```python
from build123d import *

# Parameters (mm, degrees)
SKETCH2_W                = 6
SKETCH2_H                = 14.5
BOSS_EXTRUDE1_DEPTH      = 5
SKETCH3_R                = 2.5
SKETCH3_R_2              = 1.8
BOSS_EXTRUDE2_DEPTH      = 2.5
CHAMFER2_SIZE            = 0.2
CHAMFER3_SIZE            = 0.2
SKETCH4_R                = 1.8
CUT_EXTRUDE1_DEPTH       = 14.02
SKETCH5_R                = 0.75
BOSS_EXTRUDE3_DEPTH      = 0.75
FILLET1_R                = 0.2
SKETCH7_W                = 0.344908333
SKETCH7_H                = 1.981698852
CUT_EXTRUDE2_DEPTH       = 12.710038429
SURFACE_EXTRUDE1_1_BACK  = 0.5
SURFACE_EXTRUDE1_1_DEPTH = 1
THICKEN1_T1              = 0.1
SKETCH9_W                = 1
SKETCH9_H                = 0.1
BOSS_EXTRUDE4_DEPTH      = 0.961518788
SURFACE_EXTRUDE2_2_BACK  = 0.5
SURFACE_EXTRUDE2_2_DEPTH = 1
THICKEN2_T2              = 0.1
SKETCH11_W               = 1.821073917
SKETCH11_H               = 5.660094607
CUT_EXTRUDE3_DEPTH       = 2


with BuildPart() as part:
    # Sketch2 → Boss-Extrude1 (new body)
    with BuildSketch(Plane(origin=(0, 0, 0), x_dir=(1, 0, 0), z_dir=(0, 1, 0))):
        Rectangle(SKETCH2_W, SKETCH2_H)
    extrude(amount=BOSS_EXTRUDE1_DEPTH)

    # Sketch3 → Boss-Extrude2 (add)
    with BuildSketch(Plane.XY.offset(7.25)):
        with Locations(Location((0, 2.5, 0), (0, 0, 270))):
            Circle(SKETCH3_R)
        with Locations((0, 2.5)):
            Circle(SKETCH3_R_2, mode=Mode.SUBTRACT)
    extrude(amount=BOSS_EXTRUDE2_DEPTH)

    # Chamfer2
    chamfer2_edges = [part.edges().sort_by_distance(p)[0] for p in [
        (0, 5, 9.75),
    ]]
    chamfer(chamfer2_edges, length=CHAMFER2_SIZE)

    # Chamfer3
    chamfer3_edges = [part.edges().sort_by_distance(p)[0] for p in [
        (-1.8, 2.5, 9.75),
    ]]
    chamfer(chamfer3_edges, length=CHAMFER3_SIZE)

    # Sketch4 → Cut-Extrude1 (cut)
    with BuildSketch(Plane.XY.offset(7.25)):
        with Locations((0, 2.5)):
            Circle(SKETCH4_R)
    extrude(amount=-CUT_EXTRUDE1_DEPTH, mode=Mode.SUBTRACT)

    # Sketch5 → Boss-Extrude3 (add)
    with BuildSketch(Plane.XZ):
        with Locations(Location((0, 4.191398765, 0), (0, 0, 90))):
            Circle(SKETCH5_R)
        with Locations(Location((0, -3.600413433, 0), (0, 0, 90))):
            Circle(SKETCH5_R)
    extrude(amount=BOSS_EXTRUDE3_DEPTH)

    # Fillet1
    fillet1_edges = [part.edges().sort_by_distance(p)[0] for p in [
        (0, -0.75, 3.441398765),
        (0, -0.75, -4.350413433),
    ]]
    fillet(fillet1_edges, radius=FILLET1_R)

    # Sketch7 → Cut-Extrude2 (cut, through all)
    with BuildSketch(Plane(origin=(0, 5, 0), x_dir=(1, 0, 0), z_dir=(0, 1, 0))):
        with Locations((2.827545834, -5.146058424)):
            Rectangle(SKETCH7_W, SKETCH7_H)
    extrude(amount=-CUT_EXTRUDE2_DEPTH, mode=Mode.SUBTRACT)

    # Surface-Extrude1: a surface, the sketch's curves swept straight by 1 mm
    with BuildLine(Plane.XY.offset(5.1).offset(-SURFACE_EXTRUDE1_1_BACK), mode=Mode.PRIVATE) as surface_extrude1_1_path:
        Line((2.555091667, 0.638024488), (2.555091667, 0.294273869))
        ThreePointArc((2.555091667, 0.294273869), (2.641282487, 0.086190821), (2.849365536, 0))
        Line((2.849365536, 0), (3.961518788, 0))
    surface_extrude1_1 = Shell.extrude(surface_extrude1_1_path.wire(), (0 * SURFACE_EXTRUDE1_1_DEPTH, 0 * SURFACE_EXTRUDE1_1_DEPTH, 1 * SURFACE_EXTRUDE1_1_DEPTH))
    add(Solid.thicken(surface_extrude1_1, THICKEN1_T1))

    # Sketch9 → Boss-Extrude4 (add)
    with BuildSketch(Plane(origin=(3, 0, 0), x_dir=(0, 0, -1), z_dir=(1, 0, 0))):
        with Locations((4.604659924, 0.05)):
            Rectangle(SKETCH9_W, SKETCH9_H)
    extrude(amount=BOSS_EXTRUDE4_DEPTH)

    # Surface-Extrude2: a surface, the sketch's curves swept straight by 1 mm
    with BuildLine(Plane.ZY.offset(-SURFACE_EXTRUDE2_2_BACK), mode=Mode.PRIVATE) as surface_extrude2_2_path:
        Line((-7.25, 2.862656565), (-7.25, 0.652010512))
        ThreePointArc((-7.25, 0.652010512), (-7.440969458, 0.190969458), (-7.902010512, 0))
        Line((-7.902010512, 0), (-9.009741204, 0))
    surface_extrude2_2 = Shell.extrude(surface_extrude2_2_path.wire(), (-1 * SURFACE_EXTRUDE2_2_DEPTH, 0 * SURFACE_EXTRUDE2_2_DEPTH, 0 * SURFACE_EXTRUDE2_2_DEPTH))
    add(Solid.thicken(surface_extrude2_2, -THICKEN2_T2))

    # Sketch11 → Cut-Extrude3 (cut)
    with BuildSketch(Plane.ZY.offset(3)):
        with Locations((3.036115989, 3.2980341)):
            Rectangle(SKETCH11_W, SKETCH11_H)
    extrude(amount=-CUT_EXTRUDE3_DEPTH, mode=Mode.SUBTRACT)


solid = part.part
```
Geometry check sheet. Reference: the model listing, model coordinates, mm. A direction names the side the tool comes from. Give positions to 0.01 mm unless a question says otherwise; leave off trailing zeros. Write each loop counter-clockwise with the first axis right and the second up, starting at its lowest first coordinate (ties: lowest second). Pieces come first, ordered by that corner, then holes.
1) Gauge pin test, flat ends, axial feed: pin 1 (1.5 mm diameter, centred on y = 1.5, z = -2, fed in from +X); pin 2 (0.5 mm diameter, centred on x = 3.5, z = 5, fed in from -Y); pin 3 (0.9 mm diameter, centred on y = 1, z = -8, fed in from -X); pin 4 (1.8 mm diameter, centred on x = 0, y = 2, fed in from +Z). Record the tip position at first contact, or that the pin passes through.
2) Section check B-B, the plane x = 3.25. Record the boundary of the cut face in (y, z).
3) Release check for a two-part mould opening along Y. For faces 1 (the flat face through (0, 5, 0)), 2 (the flat face through (0, 3, -6.77)), 3 (the flat face through (0, 2, -7.35)) record: pulls with the +Y half, pulls with the -Y half, needs draft (parallel to the pull), parting line crosses it, or undercut.
4) Access from +Z, -Z, +X, -X, +Y, -Y to the whole of each face (thin tool, end or side, straight path). Record for faces 4 (the flat face through (-2, 3, 2.126)), 5 (the cylindrical face through (0.751, 0.115, 8.384)), 6 (the flat face through (-3, 2, 0)).
5) Section check C-C, the plane y = 2.5. Record the boundary of the cut face in (x, z).
6) Section check A-A, the plane z = 2.5. Record the boundary of the cut face in (x, y).
7) Material ranges on L1, parallel to Y at x = 0, z = 3; L2, parallel to Z at x = 0, y = 2; L3, parallel to Z at x = 2.75, y = 2.9, recorded low to high.
Computed:
1. pin 1: stops at x = 3
1. pin 2: stops at y = 0
1. pin 3: passes through
1. pin 4: stops at z = -6.77
2. outline: (0, -5.1) - (0.1, -5.1) - (0.1, -4.1) - (0, -4.1) - close; (0, 4.6) - (0.1, 4.6) - (0.1, 5.6) - (0, 5.6) - close
3. face 1: pulls with the +Y half
3. face 2: undercut
3. face 3: needs draft
4. face 4: -X, +Y
4. face 5: +Z
4. face 6: +Z, -Z, -X, +Y, -Y
5. outline: (-3, -7.25) - (-0.5, -7.25) - (-0.5, -7.35) - (0.5, -7.35) - (0.5, -7.25) - (3, -7.25) - (3, 4.16) - (2.66, 4.16) - (2.66, 6.14) - (3, 6.14) - (3, 7.25) - (2.5, 7.25) - (2.5, 9.55) - (2.3, 9.75) - (2, 9.75) - (1.8, 9.55) - (1.8, -6.77) - (-1.8, -6.77) - (-1.8, 2.13) - (-3, 2.13) - close; (-3, 3.95) - (-1.8, 3.95) - (-1.8, 9.55) - (-2, 9.75) - (-2.3, 9.75) - (-2.5, 9.55) - (-2.5, 7.25) - (-3, 7.25) - close
6. outline: (-3, 0) - (3, 0) - (3, 5) - (-1, 5) - (-1, 4) arc R1.8 cw (long way) to (-1, 1) - (-1, 0.47) - (-3, 0.47) - close
7. L1: y = 0 to 0.7, 4.3 to 5
7. L2: z = -7.35 to -6.77
7. L3: z = -7.25 to 4.16, 6.14 to 7.25
